Could you check a few things on this model? Use its own coordinates, in mm. A direction names the side the tool comes from. Give positions to 0.01 mm unless a question says otherwise; leave off trailing zeros. Write each loop counter-clockwise with the first axis right and the second up, starting at its lowest first coordinate (ties: lowest second). Pieces come first, ordered by that corner, then holes. Notation, with made-up numbers: M 69,51.5 L 92,51.5 A19 cw 92,56.5 Z; hole C -32.5,10 d1. An arc over 180 degrees is marked long. Use one line per item in the form item = value.
from build123d import *

# Parameters (mm, degrees)
F1_DEPTH = 63.5
F2_DEPTH = 25.4
F3_DEPTH = 7.9375
F5_R     = 6.35


with BuildPart() as f1:
    # F0 (on Front) → F1 (new body, symmetric)
    with BuildSketch(Plane.XZ):
        Polygon((-41.275, 9.525), (-41.275, -9.525), (41.275, -9.525), (41.275, 9.525), (22.225, 9.525), align=None)
    extrude(amount=F1_DEPTH, both=True)

    # F0 (on Front) → F2 (join, symmetric)
    with BuildSketch(Plane.XZ):
        with BuildLine():
            Line((22.225, 9.525), (41.275, 9.525))
            Line((41.275, 9.525), (41.275, 27.0002))
            ThreePointArc((41.275, 27.0002), (45.92468, 38.22552), (57.15, 42.8752))
            Line((57.15, 42.8752), (60.325, 42.8752))
            Line((60.325, 42.8752), (60.325, 61.9252))
            Line((60.325, 61.9252), (57.15, 61.9252))
            add(Edge.make_bspline(
                [(55.536606, 61.887914), (56.072947, 61.901034), (56.610752, 61.913456), (57.15, 61.9252)],
                knots=[110.452417, 110.452417, 110.452417, 110.452417, 111.504536, 111.504536, 111.504536, 111.504536], degree=3))
            ThreePointArc((55.536606, 61.887914), (31.890315, 51.118739), (22.225, 27.0002))
            Line((22.225, 27.0002), (22.225, 9.525))
        make_face()
        Polygon((85.725, 61.9252), (60.325, 61.9252), (60.325, 42.8752), (60.325, 38.1), (85.725, 38.1), align=None)
    extrude(amount=F2_DEPTH, both=True)

    # F0 (on Front) → F3 (join, symmetric)
    with BuildSketch(Plane.XZ):
        with BuildLine():
            add(Edge.make_bspline(
                [(-41.275, 9.525), (-40.940461, 51.429681), (-0.768926, 60.510521), (55.536606, 61.887914)],
                knots=[0, 0, 0, 0, 110.452417, 110.452417, 110.452417, 110.452417], degree=3))
            Line((-41.275, 9.525), (22.225, 9.525))
            Line((22.225, 9.525), (22.225, 27.0002))
            ThreePointArc((22.225, 27.0002), (31.890315, 51.118739), (55.536606, 61.887914))
        make_face()
    extrude(amount=F3_DEPTH, both=True)

    # F0 (on Front) → F4 (revolve)
    with BuildSketch(Plane.XZ):
        Polygon((85.725, 66.675), (85.725, 61.9252), (85.725, 38.1), (111.125, 38.1), (111.125, 66.675), align=None)
    revolve(axis=Axis((85.725, 0, 52.3875), (0, 0, 1)))

    # F5
    f5_edges = [f1.edges().sort_by_distance(p)[0] for p in [
        (41.275, -63.5, 0),
        (-41.275, -63.5, 0),
        (41.275, 63.5, 0),
        (-41.275, 63.5, 0),
    ]]
    fillet(f5_edges, radius=F5_R)


solid = f1.part
1) I want a section at C-C, the plane x = 101. Please give me the cut outline in (y, z) (3 decimals).
Checked values:
outline = M -20.294,38.1 L 20.294,38.1 L 20.294,66.675 L -20.294,66.675 Z
2) I want a section at A-A, the plane z = 4. Please give me the cut outline in (x, y) (3 decimals), plus the area to 3 significant figures.
Checked values:
outline = M -41.275,-57.15 A6.35 ccw -34.925,-63.5 L 34.925,-63.5 A6.35 ccw 41.275,-57.15 L 41.275,57.15 A6.35 ccw 34.925,63.5 L -34.925,63.5 A6.35 ccw -41.275,57.15 Z
area = 10,400 mm2
3) Thinking about a two-plate mould opening in X: for faces 6 (the flat face through (60.325, 0, 41)), 7 (the flat face through (-1, -1, -9.525)), 8 (the cylindrical face through (39.365, -61.689, 0.133)), which applies, released by +X, released by -X, zero draft, split by the parting line, or undercut?
Checked values:
face_6 = undercut
face_7 = zero draft
face_8 = released by +X
4) For faces 1 (the flat face through (60, -2, 61.925)), 2 (the flat face through (86, 0, 38.1)), 3 (the flat face through (46, -25.4, 42)), 4 (the flat face through (1, -36, 9.525)), 5 (the cylindrical face through (109.95, 7.63, 55.76)), which set-ups out of +Z, -Z, +X, -X, +Y, -Y let a thin tool reach every point of the face, with its end or its side?
Checked values:
face_1 = +Z, -X
face_2 = -Z, +X, +Y, -Y
face_3 = +Z, +X, -X, -Y
face_4 = +Z, -X, -Y
face_5 = +Z
5) I want a section at B-B, the plane y = -49. Please give me the cut outline in (x, z) (3 decimals).
Checked values:
outline = M -41.275,-9.525 L 41.275,-9.525 L 41.275,9.525 L -41.275,9.525 Z
6) For pin 1 Ø5 at (x, z) = (2, 35) entering from -Y; pin 2 Ø2 at (x, z) = (-17, 15.5) entering from +Y; pin 3 Ø2.5 at (x, y) = (58.5, -10) entering from -Z, each with a flat end and sliding along its axis, tell me the tip position at first contact or that it passes through.
Checked values:
pin_1 = -7.94
pin_2 = 7.94
pin_3 = 42.88
7) If I drill on L1, parallel to Z at x = -18.5, y = 18 (3 decimals); L2, parallel to Y at x = -15, z = 29; L3, parallel to Y at x = 86, z = 44, over which ranges is the centre line in solid material (lowest first)?
Checked values:
L1 = -9.525 to 9.525
L2 = -7.94 to 7.94
L3 = -25.4 to 25.4
